from build123d import *

# Parameters (mm, degrees)
BOSS_EXTRUDE1_DEPTH = 37.338
SKETCH3_R           = 5.596968057
CUT_EXTRUDE1_DEPTH  = 37.338


with BuildPart() as part:
    # Sketch2 → Boss-Extrude1 (new body)
    with BuildSketch(Plane.XY):
        Polygon((-33.242470299, 19.191529245), (-18.64445456, 19.191529245), (-18.64445456, -0.593055445), (3.910861921, -0.593055445), (3.910861921, -5.927055445), (1.768214677, -2.879055445), (-20.93045456, -2.879055445), (-20.93045456, 16.905529245), (-36.39768935, 16.905529245), align=None)
    extrude(amount=-BOSS_EXTRUDE1_DEPTH)

    # Sketch3 → Cut-Extrude1 (cut)
    with BuildSketch(Plane(origin=(0, -0.593055445, 0), x_dir=(1, 0, 0), z_dir=(0, 1, 0))):
        with Locations(Location((-7.36679632, 18.669, 0), (0, 0, 180))):
            Circle(SKETCH3_R)
    extrude(amount=-CUT_EXTRUDE1_DEPTH, mode=Mode.SUBTRACT)


solid = part.part
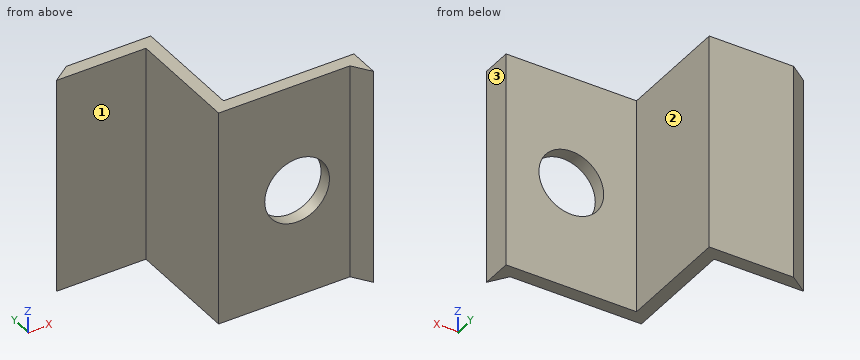
Design review of the part built by this model. Coordinates are the model's own, in mm. Face numbers are marked on the shaded views. A direction names the side the tool comes from. Coordinates: 2 decimals unless noted, no trailing zeros. Loops run counter-clockwise (first coordinate to the right, second up) from the corner with the lowest first, then second, coordinate; pieces in that order, holes last.
Item 1: Wall thickness on L1, parallel to Y at x = -29.5, z = -16.5; L2, parallel to Y at x = -14.5, z = -14.5; L3, parallel to X at y = 9.75, z = -29: over which ranges is each line inside the solid? List them lowest first.
Completed:
L1: y = 16.91 to 19.19
L2: y = -2.88 to -0.59
L3: x = -20.93 to -18.64
Item 2: For the marked faces 1, 2 and 3, list the 3-axis set-ups (+Z, -Z, +X, -X, +Y, -Y) from which the entire face can be reached by the end or side of a thin tool; tool diameter is ignored.
Completed:
face 1: +Z, -Z, -X, -Y
face 2: +Z, -Z, +X, +Y
face 3: +Z, -Z, +X, +Y, -Y
Item 3: Add section A-A (x = -6). Write out the cut boundary in (y, z), and give its area (3 significant figures).
Completed:
outline: (-2.88, -37.34) - (-0.59, -37.34) - (-0.59, -24.1) - (-2.88, -24.1) - close; (-2.88, -13.24) - (-0.59, -13.24) - (-0.59, 0) - (-2.88, 0) - close
area: 60.5 mm2
Item 4: Add section C-C (z = -28). Write out the cut boundary in (x, y), and give its area (3 significant figures).
Completed:
outline: (-36.4, 16.91) - (-20.93, 16.91) - (-20.93, -2.88) - (1.77, -2.88) - (3.91, -5.93) - (3.91, -0.59) - (-18.64, -0.59) - (-18.64, 19.19) - (-33.24, 19.19) - close
area: 137 mm2
Item 5: Add section B-B (z = -14). Write out the cut boundary in (x, y), and give its area (3 significant figures).
Completed:
outline: (-36.4, 16.91) - (-20.93, 16.91) - (-20.93, -2.88) - (-10.45, -2.88) - (-10.45, -0.59) - (-18.64, -0.59) - (-18.64, 19.19) - (-33.24, 19.19) - close; (-4.28, -2.88) - (1.77, -2.88) - (3.91, -5.93) - (3.91, -0.59) - (-4.28, -0.59) - close
area: 123 mm2
Item 6: Clearance check with flat-ended pins moving along their axes: pin 1 (18 mm diameter, centred on x = -7.37, z = -18.67, fed in from -Y); pin 2 (1 mm diameter, centred on y = -1.5, z = -29.5, fed in from -X); pin 3 (1.5 mm diameter, centred on x = -3.5, z = -4, fed in from +Y). State where each tip first meets the part, or that it passes through.
Completed:
pin 1: stops at y = -2.88
pin 2: stops at x = -20.93
pin 3: stops at y = -0.59
Item 7: Add section D-D (y = -2). Write out the cut boundary in (x, z), and give its area (3 significant figures).
Completed:
outline: (-20.93, -37.34) - (3.91, -37.34) - (3.91, 0) - (-20.93, 0) - close; hole circle Ø11.19 at (-7.37, -18.67)
area: 829 mm2
